```python
from build123d import *

# Parameters (mm, degrees)
SKETCH1_W           = 20
SKETCH1_H           = 6
BOSS_EXTRUDE1_DEPTH = 6


with BuildPart() as part:
    # Sketch1 → Boss-Extrude1 (new body)
    # profile 1 of 3: a face of its own
    with BuildSketch(Plane.XY):
        with BuildLine():
            ThreePointArc((27.5, 45), (38.106601718, 40.606601718), (42.5, 30))
            Line((42.5, 30), (42.5, -30.857864376))
            ThreePointArc((42.5, -30.857864376), (39.747448714, -39.518118414), (32.5, -45))
            Line((32.5, -45), (-27.5, -45))
            ThreePointArc((-27.5, -45), (-38.106601718, -40.606601718), (-42.5, -30))
            Line((-42.5, -30), (-42.5, 30))
            ThreePointArc((-42.5, 30), (-38.106601718, 40.606601718), (-27.5, 45))
            Line((-27.5, 45), (27.5, 45))
        make_face()
        with BuildLine():
            ThreePointArc((27.5, -33.112673684), (30.612673684, -30), (27.5, -26.887326316))
            Line((27.5, -26.887326316), (-27.5, -26.887326316))
            ThreePointArc((-27.5, -26.887326316), (-30.612673684, -30), (-27.5, -33.112673684))
            Line((-27.5, -33.112673684), (27.5, -33.112673684))
        make_face(mode=Mode.SUBTRACT)
        with BuildLine():
            ThreePointArc((27.5, -23.112673684), (30.612673684, -20), (27.5, -16.887326316))
            Line((27.5, -16.887326316), (-27.5, -16.887326316))
            ThreePointArc((-27.5, -16.887326316), (-30.612673684, -20), (-27.5, -23.112673684))
            Line((-27.5, -23.112673684), (27.5, -23.112673684))
        make_face(mode=Mode.SUBTRACT)
        with BuildLine():
            ThreePointArc((27.5, -13.112673684), (30.612673684, -10), (27.5, -6.887326316))
            Line((27.5, -6.887326316), (-27.5, -6.887326316))
            ThreePointArc((-27.5, -6.887326316), (-30.612673684, -10), (-27.5, -13.112673684))
            Line((-27.5, -13.112673684), (27.5, -13.112673684))
        make_face(mode=Mode.SUBTRACT)
        with BuildLine():
            ThreePointArc((27.5, -3.112673684), (30.612673684, 0), (27.5, 3.112673684))
            Line((27.5, 3.112673684), (-27.5, 3.112673684))
            ThreePointArc((-27.5, 3.112673684), (-30.612673684, 0), (-27.5, -3.112673684))
            Line((-27.5, -3.112673684), (27.5, -3.112673684))
        make_face(mode=Mode.SUBTRACT)
        with BuildLine():
            ThreePointArc((27.5, 6.887326316), (30.612673684, 10), (27.5, 13.112673684))
            Line((27.5, 13.112673684), (-27.5, 13.112673684))
            ThreePointArc((-27.5, 13.112673684), (-30.612673684, 10), (-27.5, 6.887326316))
            Line((-27.5, 6.887326316), (27.5, 6.887326316))
        make_face(mode=Mode.SUBTRACT)
        with BuildLine():
            ThreePointArc((27.5, 16.887326316), (30.612673684, 20), (27.5, 23.112673684))
            Line((27.5, 23.112673684), (-27.5, 23.112673684))
            ThreePointArc((-27.5, 23.112673684), (-30.612673684, 20), (-27.5, 16.887326316))
            Line((-27.5, 16.887326316), (27.5, 16.887326316))
        make_face(mode=Mode.SUBTRACT)
        with BuildLine():
            ThreePointArc((27.5, 26.887326316), (30.612673684, 30), (27.5, 33.112673684))
            Line((27.5, 33.112673684), (-27.5, 33.112673684))
            ThreePointArc((-27.5, 33.112673684), (-30.612673684, 30), (-27.5, 26.887326316))
            Line((-27.5, 26.887326316), (27.5, 26.887326316))
        make_face(mode=Mode.SUBTRACT)
    # profile 2 of 3: a face of its own
    with BuildSketch(Plane.XY):
        with Locations((0, 48)):
            Rectangle(SKETCH1_W, SKETCH1_H)
    # profile 3 of 3: a face of its own
    with BuildSketch(Plane.XY):
        with Locations((0, -48)):
            Rectangle(SKETCH1_W, SKETCH1_H)
    extrude(amount=BOSS_EXTRUDE1_DEPTH)


solid = part.part
```
Work out the finished part from the listing and answer in its coordinate system (mm). A direction names the side the tool comes from. Coordinates: 2 decimals unless noted, no trailing zeros. Order: outer loops, then holes, each group sorted by start corner. A loop starts at its lowest first (then second) coordinate and runs counter-clockwise, first axis right, second up. Notation, with made-up numbers: M -33,82 L 0,82 A34 ccw 0,117 Z; hole C 34,40 d7. An arc over 180 degrees is marked long. Use CSV: the item, a comma, the result in double quotes.
1) For faces 1 (the face through (10, 48, 3)), 2 (the face through (-10, 48, 3)), 3 (the face through (30.61, 19.93, 2.96)), determine the directions among +Z, -Z, +X, -X, +Y, -Y from which every point of the face is accessible in a straight line to the end or side of a thin tool.
Worked out:
face 1,"+Z, -Z, +X, +Y"
face 2,"+Z, -Z, -X, +Y"
face 3,"+Z, -Z"
2) Section B-B on x = 1 is taken. Count the separate pieces of the cut face and the enclosed holes in it, plus the area to 3 significant figures.
Worked out:
separate pieces,"8"
enclosed holes,"0"
area,"351 mm^2"
3) Flat-ended cylindrical pins translate along their axes: pin 1 Ø1.8 at (x, z) = (12.5, 3.5) entering from -Y; pin 2 Ø3 at (x, z) = (10.5, 4) entering from -Y; pin 3 Ø3 at (x, z) = (-23, 4) entering from +Y; pin 4 Ø3 at (y, z) = (-49, 2) entering from +X. Find the tip coordinate at first contact, or state that the pin passes through.
Worked out:
pin 1,"stops at y = -45"
pin 2,"stops at y = -51"
pin 3,"stops at y = 45"
pin 4,"stops at x = 10"
4) Section D-D on y = -18 is taken. Write down the section's boundary in (x, z).
Worked out:
outline,"M -42.5,0 L -29.89,0 L -29.89,6 L -42.5,6 Z; M 29.89,0 L 42.5,0 L 42.5,6 L 29.89,6 Z"
5) Determine the mould class of faces 4 (the face through (-38.22, 40.49, 2.96)), 5 (the face through (0, 13.113, 3)), 6 (the face through (0.6, 23.4, 0)) for opening direction X: released by +X, released by -X, zero draft, split by the parting line, or undercut.
Worked out:
face 4,"released by -X"
face 5,"undercut"
face 6,"zero draft"
6) Consider line 1 (X direction, y = 27.5, z = 1.9); line 2 (X direction, y = 20.5, z = 3.65); line 3 (X direction, y = -36.5, z = 2.1). Determine where each line is inside the solid, lowest interval first. Write a range as [from, to].
Worked out:
line 1,"x = [-42.5, -29.35], [29.35, 42.5]"
line 2,"x = [-42.5, -30.57], [30.57, 42.5]"
line 3,"x = [-41.02, 41.4]"
7) Section A-A on y = 20 is taken. Write down the section's boundary in (x, z), plus the area to 3 significant figures.
Worked out:
outline,"M -42.5,0 L -30.61,0 L -30.61,6 L -42.5,6 Z; M 30.61,0 L 42.5,0 L 42.5,6 L 30.61,6 Z"
area,"143 mm^2"
